For this review, take the finished solid that the model builds, in its own axes (mm). A direction names the side the tool comes from. Coordinates: 2 decimals unless noted, no trailing zeros. Order: outer loops, then holes, each group sorted by start corner. A loop starts at its lowest first (then second) coordinate and runs counter-clockwise, first axis right, second up. Notation, with made-up numbers: M 71.25,15.25 L 112.25,15.25 A8 ccw 112.25,19.25 Z; hole C 39.5,27.25 d4. An arc over 180 degrees is marked long. Use CSV: the item, a comma, the result in double quotes.
```python
from build123d import *

# Parameters (mm, degrees)
F0_W     = 139.7
F0_H     = 101.6
F1_DEPTH = 6.35
F2_W     = 29.21
F2_H     = 10.16
F2_W_2   = 10.795
F3_DEPTH = 25.4
F5_R     = 2.0955
F6_DEPTH = 25.4
F7_W     = 6.35
F7_H     = 25.4
F8_DEPTH = 25.4


with BuildPart() as f1:
    # F0 (on Top) → F1 (new body)
    with BuildSketch(Plane.XY):
        with Locations((69.85, -50.8)):
            Rectangle(F0_W, F0_H)
    extrude(amount=F1_DEPTH)

    # F2 (on face) → F3 (cut)
    with BuildSketch(Plane.XY.offset(6.35)):
        with Locations((55.245, -45.72)):
            Rectangle(F2_W, F2_H)
        with Locations((75.2475, -45.72)):
            Rectangle(F2_W_2, F2_H)
        with Locations((55.245, -55.88)):
            Rectangle(F2_W, F2_H)
        with Locations((75.2475, -55.88)):
            Rectangle(F2_W_2, F2_H)
    extrude(amount=-F3_DEPTH, mode=Mode.SUBTRACT)

    # F5 (on face) → F6 (cut)
    with BuildSketch(Plane.XY.offset(6.35)):
        with Locations((84.7725, -45.085)):
            Circle(F5_R)
        with Locations((84.7725, -56.515)):
            Circle(F5_R)
        with Locations((36.5125, -45.085)):
            Circle(F5_R)
        with Locations((36.5125, -56.515)):
            Circle(F5_R)
    extrude(amount=-F6_DEPTH, mode=Mode.SUBTRACT)

    # F7 (on face) → F8 (cut)
    with BuildSketch(Plane.XY.offset(6.35)):
        with Locations((3.175, -25.4)):
            Rectangle(F7_W, F7_H)
        with Locations((3.175, -76.2)):
            Rectangle(F7_W, F7_H)
        with Locations((136.525, -25.4)):
            Rectangle(F7_W, F7_H)
        with Locations((136.525, -76.2)):
            Rectangle(F7_W, F7_H)
    extrude(amount=-F8_DEPTH, mode=Mode.SUBTRACT)


solid = f1.part
```
Item 1: Add section A-A on z = 2.5. State how many separate pieces and enclosed holes the cut face has, and give its area (3 significant figures).
Solutions:
separate pieces,"1"
enclosed holes,"5"
area,"12,700 mm^2"
Item 2: For faces 4 (the face through (139.7, -51, 3)), 5 (the face through (133.35, -26, 3)), 6 (the face through (40.64, -51, 3)), 7 (the face through (3, -38.1, 3)), list the 3-axis set-ups (+Z, -Z, +X, -X, +Y, -Y) from which the entire face can be reached by the end or side of a thin tool; tool diameter is ignored.
Solutions:
face 4,"+Z, -Z, +X, +Y, -Y"
face 5,"+Z, -Z, +X"
face 6,"+Z, -Z"
face 7,"+Z, -Z, -X"
Item 3: Clearance check with flat-ended pins moving along their axes: pin 1 Ø3 at (y, z) = (-74, 2.5) entering from +X; pin 2 Ø1.9 at (y, z) = (-23.5, 2.5) entering from -X; pin 3 Ø3.5 at (x, y) = (84.77, -45.08) entering from -Z. State where each tip first meets the part, or that it passes through.
Solutions:
pin 1,"x = 133.35"
pin 2,"x = 6.35"
pin 3,"through"
Item 4: Add section B-B on y = -73.5. State the section outline as (x, z) points.
Solutions:
outline,"M 6.35,0 L 133.35,0 L 133.35,6.35 L 6.35,6.35 Z"
Item 5: To check wall thickness, follow line 1 along X through (y, z) = (-60, 2.25) (3 decimals); line 2 along X through (y, z) = (-46.5, 5.5) (3 decimals); line 3 along Y through (x, z) = (68, 5.75). State the ranges of each line that lie inside material, in increasing order. Write a range as [from, to].
Solutions:
line 1,"[0, 40.64], [80.645, 139.7]"
line 2,"[0, 34.967], [38.058, 40.64], [80.645, 83.227], [86.318, 139.7]"
line 3,"[-101.6, -60.96], [-40.64, 0]"
Item 6: Draft analysis for pull direction X (two halves, no side actions). For faces 1 (the face through (60, -60.96, 3)), 2 (the face through (139.7, -95, 3)), 3 (the face through (0, -51, 3)), state which applies: released by +X, released by -X, zero draft, split by the parting line, or undercut.
Solutions:
face 1,"undercut"
face 2,"released by +X"
face 3,"released by -X"
